Check sheet for the drawn part. Datum: minimum x, y, z corner. Units: mm. A direction names the side the tool comes from. Round coordinates to 2 decimals unless told otherwise and drop trailing zeros. Write each loop counter-clockwise with the first axis right and the second up, starting at its lowest first coordinate (ties: lowest second). Pieces come first, ordered by that corner, then holes.
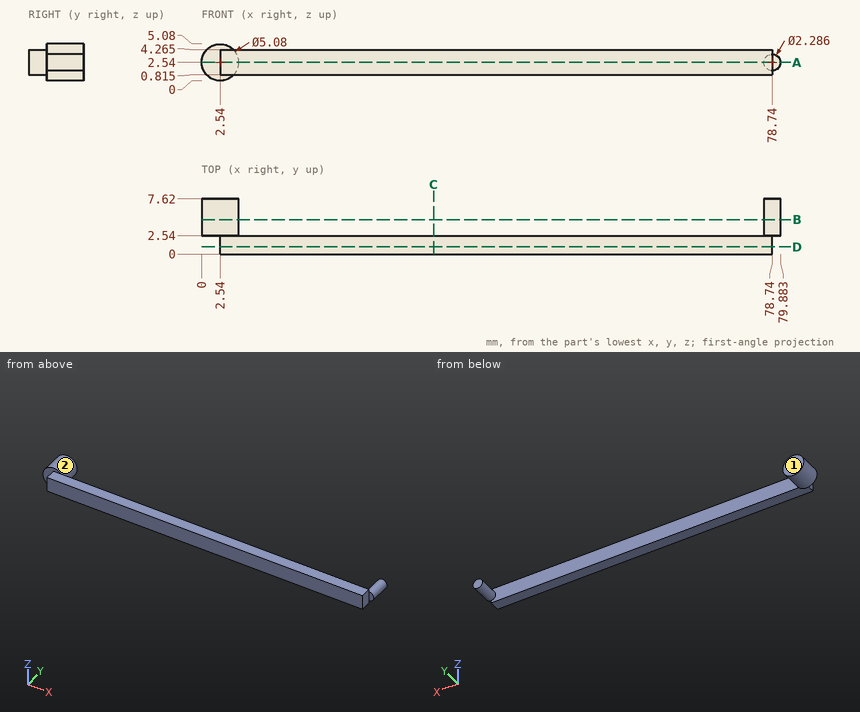
Q1. Sectioned sample at D-D (y = 1). Enter the section's corners in (x, z) (1 decimal).
Recorded:
outline: (2.5, 0.8) - (78.7, 0.8) - (78.7, 4.3) - (2.5, 4.3) - close
Q2. Sectioned sample at A-A (z = 2.54). Enter the section's corners in (x, y).
Recorded:
outline: (0, 2.54) - (2.54, 2.54) - (2.54, 0) - (78.74, 0) - (78.74, 2.54) - (79.88, 2.54) - (79.88, 7.62) - (77.6, 7.62) - (77.6, 2.54) - (5.08, 2.54) - (5.08, 7.62) - (0, 7.62) - close
Q3. Depth check by flat-ended pin: P1, Ø2, axis at x = 30, z = 4.5, coming from the +Y side; P2, Ø3, axis at x = 29.5, y = 1, coming from the -Z side (1 decimal); P3, Ø1.3, axis at y = 1.5, z = 2, coming from the +X side; P4, Ø1, axis at x = 63, y = 3.5, coming from the -Z side. Enter the tip coordinate at first touch or a pass-through.
Recorded:
P1: stops at y = 2.54
P2: stops at z = 0.8
P3: stops at x = 78.74
P4: passes through
Q4. Material ranges on line 1 along X through (y, z) = (3.25, 2.55); line 2 along Z through (x, y) = (71.5, 2) (1 decimal); line 3 along X through (y, z) = (1.25, 2.45), recorded low to high.
Recorded:
line 1: x = 0 to 5.08, 77.6 to 79.88
line 2: z = 0.8 to 4.3
line 3: x = 2.54 to 78.74
Q5. Tool access check on the marked faces 1 and 2. Record the directions out of +Z, -Z, +X, -X, +Y, -Y that give a thin tool (end or side, any length) a straight path to the whole face; none if there is none.
Recorded:
face 1: +Z, -Z, +X, -X, +Y
face 2: +Y
Q6. Sectioned sample at C-C (x = 32). Enter the section's corners in (y, z) (1 decimal).
Recorded:
outline: (0, 0.8) - (2.5, 0.8) - (2.5, 4.3) - (0, 4.3) - close
Q7. Sectioned sample at B-B (y = 4.75). Enter the section's corners in (x, z).
Recorded:
outline: circle Ø5.08 at (2.54, 2.54); circle Ø2.29 at (78.74, 2.54)
